Build history of the part. All positions in model axes, mm. A direction names the side the tool comes from. Give positions to 0.01 mm unless a question says otherwise; leave off trailing zeros. Order: outer loops, then holes, each group sorted by start corner. A loop starts at its lowest first (then second) coordinate and runs counter-clockwise, first axis right, second up. Notation, with made-up numbers: M -29,36 L 15,36 A31 cw 15,64 Z; hole C 9.5,50.5 d2. An arc over 180 degrees is marked long. Answer as CSV lines item,"result".
from build123d import *

# Parameters (mm, degrees)
F1_DEPTH = 101.6
F3_DEPTH = 50.8
F4_W     = 25.4
F4_H     = 7.2853491507
F5_DEPTH = 21.59
F7_R     = 0.79375
F8_DEPTH = 25.4


# Not quite as in the source:
# - a feature names something its author has since deleted; it is built from what else it names


with BuildPart() as f1:
    # F0 (on Front) → F1 (new body)
    with BuildSketch(Plane.XZ):
        Polygon((50.8, 31.75), (0, 31.75), (6.35, 0), (44.45, 0), align=None)
        Polygon((44.45, 0), (6.35, 0), (0, -6.35), (50.8, -6.35), align=None)
    extrude(amount=F1_DEPTH)

    # F2 (on Right) → F3 (cut)
    with BuildSketch(Plane.YZ):
        Polygon((-101.6, 31.75), (-101.6, 19.05), (0, 31.75), align=None)
    extrude(amount=F3_DEPTH, mode=Mode.SUBTRACT)

    # F4 (on face) → F5 (cut)
    with BuildSketch(Plane.XZ.offset(101.6)):
        with Locations((26.035, 22.6926745754)):
            Rectangle(F4_W, F4_H)
        with BuildLine():
            Line((13.335, 19.05), (13.335, 7.2853491507))
            ThreePointArc((13.335, 7.2853491507), (15.9808333333, -0.6521508493), (22.86, -5.4146508493))
            Line((22.86, -5.4146508493), (29.21, -5.4146508493))
            ThreePointArc((29.21, -5.4146508493), (36.0891666667, -0.6521508493), (38.735, 7.2853491507))
            Line((38.735, 7.2853491507), (38.735, 19.05))
            Line((38.735, 19.05), (13.335, 19.05))
        make_face()
    extrude(amount=-F5_DEPTH, mode=Mode.SUBTRACT)

    # F7 (on offset) → F8 (cut, symmetric)
    with BuildSketch(Plane.YZ.offset(26.035)):
        with Locations((-101.6, -4.5212)):
            Circle(F7_R)
    extrude(amount=F8_DEPTH, both=True, mode=Mode.SUBTRACT)


solid = f1.part
Item 1: Probe line 1 along Y through (x, z) = (18.5, 21.5); line 2 along Z through (x, y) = (20, -20.5); line 3 along Z through (x, y) = (17, -71) (3 decimals). List the from-to ranges inside material, lowest first. Write a range as from..to.
Geometry says:
line 1,"y = -80.01..0"
line 2,"z = -6.35..29.19"
line 3,"z = -6.35..22.875"
Item 2: Band-saw the part on A-A (x = 45.5). Give the cut face in (y, z).
Geometry says:
outline,"M -101.6,-6.35 L 0,-6.35 L 0,-1.05 L -101.6,-1.05 L -101.6,-3.73 A0.79 cw -101.6,-5.31 Z; M -101.6,5.25 L 0,5.25 L 0,31.75 L -101.6,19.05 Z"
Item 3: 3-axis set-ups, long thin cutter, end or side, ignore diameter. For faces 5 (the flat face through (3.836, -50.089, 12.569)), 6 (the flat face through (46.875, -50.089, 12.125)), 7 (the cylindrical face through (15.91, -90.96, -0.56)): which of +Z, -Z, +X, -X, +Y, -Y reach the whole face in a straight line?
Geometry says:
face 5,"-X, +Y, -Y"
face 6,"+X, +Y, -Y"
face 7,"+Z, -Y"
Item 4: Band-saw the part on C-C (y = -82). Give the cut face in (x, z) (3 decimals).
Geometry says:
outline,"M 0,-6.35 L 50.8,-6.35 L 44.45,0 L 48.75,21.5 L 38.735,21.5 L 38.735,7.285 A13.229 cw 29.21,-5.415 L 22.86,-5.415 A13.229 cw 13.335,7.285 L 13.335,21.5 L 2.05,21.5 L 6.35,0 Z"
Item 5: Band-saw the part on B-B (x = 25.5). Give the cut face in (y, z).
Geometry says:
outline,"M -101.6,-6.35 L 0,-6.35 L 0,31.75 L -80.01,21.75 L -80.01,-5.41 L -101.6,-5.41 Z"
Item 6: Drop flat-ended pins along their axis: pin 1 (2 mm diameter, centred on y = -35, z = 14.5, fed in from -X); pin 2 (2 mm diameter, centred on y = -28.5, z = 24, fed in from -X); pin 3 (2 mm diameter, centred on x = 43, y = -13.5, fed in from +Z). Give the stop position or say it passes through.
Geometry says:
pin 1,"stops at x = 3.25"
pin 2,"stops at x = 1.35"
pin 3,"stops at z = 30.19"
Item 7: Band-saw the part on D-D (z = 20.5). Give the cut face in (x, y) (3 decimals).
Geometry says:
outline,"M 2.25,-90 L 13.335,-90 L 13.335,-80.01 L 38.735,-80.01 L 38.735,-90 L 48.55,-90 L 48.55,0 L 2.25,0 Z"
Item 8: Pull direction Z, two halves, no side cores. Call faces 1 (the flat face through (3.22, -50.09, -3.13)), 2 (the flat face through (25.04, -51.51, 25.31)), 3 (the flat face through (42, -101.6, 8)), 4 (the flat face through (47.67, -50.09, -3.22)): released by +Z, released by -Z, zero draft, split by the parting line, or undercut.
Geometry says:
face 1,"undercut"
face 2,"released by +Z"
face 3,"zero draft"
face 4,"undercut"
